from build123d import *

# Parameters (mm, degrees)
SKETCH1_R           = 0.79375
BOSS_EXTRUDE1_DEPTH = 1.27


with BuildPart() as part:
    # Sketch1 → Boss-Extrude1 (new, symmetric)
    # profile 1 of 7: a face of its own
    with BuildSketch(Plane(origin=(0, 0, 0), x_dir=(1, 0, 0), z_dir=(0, 1, 0))):
        with BuildLine():
            ThreePointArc((-4.682314967, -0.870248702), (-4.742411374, -0.436967517), (-4.7625, 0))
            ThreePointArc((-4.7625, 0), (-4.69391314, 0.805348174), (-4.490128061, 1.5875))
            Line((-4.490128061, 1.5875), (-14.2875, 1.5875))
            Line((-14.2875, 1.5875), (-14.2875, -1.5875))
            Line((-14.2875, -1.5875), (-5.924630657, -1.5875))
            Line((-5.924630657, -1.5875), (-4.682314967, -0.870248702))
        make_face()
        with Locations(Location((-11.1125, 0, 0), (0, 0, 270))):
            Circle(SKETCH1_R, mode=Mode.SUBTRACT)
    # profile 2 of 7: a face of its own
    with BuildSketch(Plane(origin=(0, 0, 0), x_dir=(1, 0, 0), z_dir=(0, 1, 0))):
        with BuildLine():
            Line((-4.7625, 0), (-3.175, 0))
            ThreePointArc((-3.175, 0), (-3.066814498, 0.821750468), (-2.749630657, 1.5875))
            Line((-2.749630657, 1.5875), (-4.490128061, 1.5875))
            ThreePointArc((-4.490128061, 1.5875), (-4.69391314, 0.805348174), (-4.7625, 0))
        make_face()
    # profile 3 of 7: a face of its own
    with BuildSketch(Plane(origin=(0, 0, 0), x_dir=(1, 0, 0), z_dir=(0, 1, 0))):
        with BuildLine():
            ThreePointArc((-2.749630657, 1.5875), (0, 3.175), (2.749630657, 1.5875))
            Line((2.749630657, 1.5875), (4.490128061, 1.5875))
            ThreePointArc((4.490128061, 1.5875), (0, 4.7625), (-4.490128061, 1.5875))
            Line((-4.490128061, 1.5875), (-2.749630657, 1.5875))
        make_face()
    # profile 4 of 7: a face of its own
    with BuildSketch(Plane(origin=(0, 0, 0), x_dir=(1, 0, 0), z_dir=(0, 1, 0))):
        with BuildLine():
            ThreePointArc((2.749630657, 1.5875), (3.066814498, 0.821750468), (3.175, 0))
            Line((3.175, 0), (4.7625, 0))
            ThreePointArc((4.7625, 0), (4.69391314, 0.805348174), (4.490128061, 1.5875))
            Line((4.490128061, 1.5875), (2.749630657, 1.5875))
        make_face()
    # profile 5 of 7: a face of its own
    with BuildSketch(Plane(origin=(0, 0, 0), x_dir=(1, 0, 0), z_dir=(0, 1, 0))):
        with BuildLine():
            ThreePointArc((4.490128061, 1.5875), (4.69391314, 0.805348174), (4.7625, 0))
            ThreePointArc((4.7625, 0), (4.742411374, -0.436967517), (4.682314967, -0.870248702))
            Line((4.682314967, -0.870248702), (5.924630657, -1.5875))
            Line((5.924630657, -1.5875), (14.2875, -1.5875))
            Line((14.2875, -1.5875), (14.2875, 1.5875))
            Line((14.2875, 1.5875), (4.490128061, 1.5875))
        make_face()
        with Locations(Location((11.1125, 0, 0), (0, 0, 270))):
            Circle(SKETCH1_R, mode=Mode.SUBTRACT)
    # profile 6 of 7: a face of its own
    with BuildSketch(Plane(origin=(0, 0, 0), x_dir=(1, 0, 0), z_dir=(0, 1, 0))):
        with BuildLine():
            Line((-4.682314967, -0.870248702), (-3.175, 0))
            Line((-3.175, 0), (-4.7625, 0))
            ThreePointArc((-4.7625, 0), (-4.742411374, -0.436967517), (-4.682314967, -0.870248702))
        make_face()
    # profile 7 of 7: a face of its own
    with BuildSketch(Plane(origin=(0, 0, 0), x_dir=(1, 0, 0), z_dir=(0, 1, 0))):
        with BuildLine():
            Line((4.7625, 0), (3.175, 0))
            Line((3.175, 0), (4.682314967, -0.870248702))
            ThreePointArc((4.682314967, -0.870248702), (4.742411374, -0.436967517), (4.7625, 0))
        make_face()
    extrude(amount=BOSS_EXTRUDE1_DEPTH, both=True)


solid = part.part
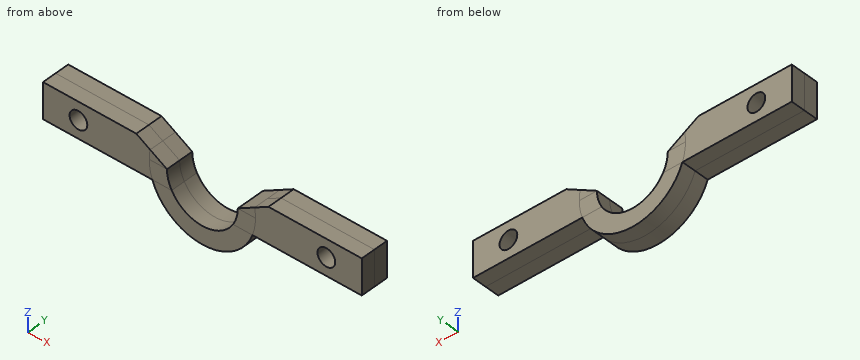
Geometry: final body of the model. Coordinates: model frame, mm. Round coordinates to 2 decimals unless told otherwise and drop trailing zeros. Loops run counter-clockwise (first coordinate to the right, second up) from the corner with the lowest first, then second, coordinate; pieces in that order, holes last. Notation, with made-up numbers: M 49,34 L 76,34 A23 cw 76,45 Z; hole C 76,-34.5 d7. An arc over 180 degrees is marked long. Put each result on its own line as item: value. Start each with the question number.
(1) Section query C-C (z = -0.25). Return loops of the section in (x, y), then the cut area to 3 significant figures.
(2) Section query A-A (z = -2.5). Return loops of the section in (x, y), then the cut area to 3 significant figures.
(3) Section query D-D (x = 6.5). Return loops of the section in (y, z).
(4) Material intervals for line 1 along Z through (x, y) = (12.5, -1.1); line 2 along X through (y, z) = (-0.05, -1.25); line 3 along X through (y, z) = (0.4, -1.75), sorted ascending. Write a range as [from, to].
(5) Contact query for a flat-ended pin moving along its axis: pin 1 Ø1.4 at (x, y) = (-11.5, 1) entering from -Z. Output: stop coordinate, or through.
(6) Section query B-B (y = -0.75). State how many separate pieces and enclosed holes the cut face has, then the cut area to 3 significant figures.
Findings below:
1. outline: M -14.29,-1.27 L -11.87,-1.27 L -11.87,1.27 L -14.29,1.27 Z; M -10.36,-1.27 L -3.17,-1.27 L -3.17,1.27 L -10.36,1.27 Z; M 3.17,-1.27 L 10.36,-1.27 L 10.36,1.27 L 3.17,1.27 Z; M 11.87,-1.27 L 14.29,-1.27 L 14.29,1.27 L 11.87,1.27 Z
1. area: 48.8 mm2
2. outline: M -4.05,-1.27 L -1.96,-1.27 L -1.96,1.27 L -4.05,1.27 Z; M 1.96,-1.27 L 4.05,-1.27 L 4.05,1.27 L 1.96,1.27 Z
2. area: 10.6 mm2
3. outline: M -1.27,-1.59 L 1.27,-1.59 L 1.27,1.59 L -1.27,1.59 Z
4. line 1: z = [-1.59, 1.59]
4. line 2: x = [-14.29, -2.92], [2.92, 14.29]
4. line 3: x = [-4.43, -2.65], [2.65, 4.43]
5. pin 1: stops at z = -1.59
6. separate pieces: 1
6. enclosed holes: 2
6. area: 77.3 mm2
